Build history of the part. All positions in model axes, mm. Coordinates: 2 decimals unless noted, no trailing zeros. Write each loop counter-clockwise with the first axis right and the second up, starting at its lowest first coordinate (ties: lowest second). Pieces come first, ordered by that corner, then holes. Notation, with made-up numbers: (62.5, 83.5) -> (109.5, 83.5) arc R29 ccw to (109.5, 121.5) -> close; hole circle Ø3 at (73.25, -3.75). An arc over 180 degrees is marked (long way). Write each question's results on one line, items separated by ' | '. Start each with the question number.
Q1. Drill centre lines: line 1 (Y direction, x = 78.5, z = 0.75); line 2 (Y direction, x = -36.5, z = 0.75); line 3 (X direction, y = 98, z = 4). Where is each one in solid material? Low to high.
Q2. Saw through at A-A on y = -14. Give the cut face in (x, z).
Q3. Saw through at B-B on x = 72.5. Give the cut face in (y, z).
Q4. Saw through at C-C on y = 35. Give the cut face in (x, z).
Q5. Two-plate mould, pull along Y, no slides. Class faces 1 (the face through (61, 25.4, 3)), 2 (the face through (139.203, 123.181, 3.131)), 3 (the face through (-139.203, -123.181, 3.131)), 4 (the face through (-90, -120.694, 3)): released by +Y, released by -Y, zero draft, split by the parting line, or undercut.
Q6. Drop flat-ended pins along their axis: pin 1 Ø3 at (y, z) = (118.5, 4) entering from +X; pin 2 Ø3 at (y, z) = (-118, 2) entering from +X; pin 3 Ø1.9 at (y, z) = (-118, 4) entering from -X. Give the stop position or say it passes through.
Q7. Saw through at D-D on x = -14. Give the cut face in (y, z).
from build123d import *

# Parameters (mm, degrees)
F0_W     = 25.4
F0_H     = 6.35
F1_DEPTH = 6.35
F2_R     = 38.1


# Not quite as in the source:
# - a feature names something its author has since deleted; it is built from what else it names


with BuildPart() as f1:
    # F0 (on Top) → F1 (new body)
    with BuildSketch(Plane.XY):
        with BuildLine():
            ThreePointArc((142.8242, 114.3), (139.1044561211, 123.2802561211), (130.1242, 127))
            Line((130.1242, 127), (-130.1242, 127))
            ThreePointArc((-130.1242, 127), (-139.1044561211, 123.2802561211), (-142.8242, 114.3))
            Line((-142.8242, 114.3), (-142.8242, -114.3))
            ThreePointArc((-142.8242, -114.3), (-139.1044561211, -123.2802561211), (-130.1242, -127))
            Line((-130.1242, -127), (130.1242, -127))
            ThreePointArc((130.1242, -127), (139.1044561211, -123.2802561211), (142.8242, -114.3))
            Line((142.8242, -114.3), (142.8242, 114.3))
        make_face()
        with Locations((-90.0851422843, -117.5192241168)):
            Rectangle(F0_W, F0_H, mode=Mode.SUBTRACT)
        with Locations((-90.0684, -3.175)):
            Rectangle(F0_W, F0_H, mode=Mode.SUBTRACT)
        with Locations((90.0851422843, -117.5192241168)):
            Rectangle(F0_W, F0_H, mode=Mode.SUBTRACT)
        with Locations((90.0684, -3.175)):
            Rectangle(F0_W, F0_H, mode=Mode.SUBTRACT)
        with Locations((-90.0851422843, 117.5192241168)):
            Rectangle(F0_W, F0_H, mode=Mode.SUBTRACT)
        with BuildLine():
            Line((0, 101.6), (7.0708802395, 101.6))
            Line((7.0708802395, 101.6), (111.125, 101.6))
            ThreePointArc((111.125, 101.6), (114.3, 104.775), (117.475, 101.6))
            ThreePointArc((117.475, 101.6), (116.5450640303, 99.3549359697), (114.3, 98.425))
            Line((114.3, 98.425), (114.3, 25.4))
            Line((114.3, 25.4), (44.3961802395, 25.4))
            Line((44.3961802395, 25.4), (37.3253, 25.4))
            Line((37.3253, 25.4), (37.3253, -25.4))
            Line((37.3253, -25.4), (44.3961802395, -25.4))
            Line((44.3961802395, -25.4), (114.3, -25.4))
            Line((114.3, -25.4), (114.3, -98.425))
            ThreePointArc((114.3, -98.425), (116.5450640303, -99.3549359697), (117.475, -101.6))
            ThreePointArc((117.475, -101.6), (114.3, -104.775), (111.125, -101.6))
            Line((111.125, -101.6), (7.0708802395, -101.6))
            Line((7.0708802395, -101.6), (0, -101.6))
            Line((0, -101.6), (-7.0708802395, -101.6))
            Line((-7.0708802395, -101.6), (-111.125, -101.6))
            ThreePointArc((-111.125, -101.6), (-116.5450640303, -103.8450640303), (-114.3, -98.425))
            Line((-114.3, -98.425), (-114.3, -25.4))
            Line((-114.3, -25.4), (-44.3961802395, -25.4))
            Line((-44.3961802395, -25.4), (-37.3253, -25.4))
            Line((-37.3253, -25.4), (-37.3253, 25.4))
            Line((-37.3253, 25.4), (-44.3961802395, 25.4))
            Line((-44.3961802395, 25.4), (-114.3, 25.4))
            Line((-114.3, 25.4), (-114.3, 98.425))
            ThreePointArc((-114.3, 98.425), (-116.5450640303, 103.8450640303), (-111.125, 101.6))
            Line((-111.125, 101.6), (-7.0708802395, 101.6))
            Line((-7.0708802395, 101.6), (0, 101.6))
        make_face(mode=Mode.SUBTRACT)
        with Locations((90.0851422843, 117.5192241168)):
            Rectangle(F0_W, F0_H, mode=Mode.SUBTRACT)
        Polygon((-37.3253, 25.4), (0, 101.6), (-7.0708802395, 101.6), (-44.3961802395, 25.4), align=None)
        Polygon((44.3961802395, 25.4), (7.0708802395, 101.6), (0, 101.6), (37.3253, 25.4), align=None)
        Polygon((44.3961802395, -25.4), (37.3253, -25.4), (0, -101.6), (7.0708802395, -101.6), align=None)
        Polygon((0, -101.6), (-37.3253, -25.4), (-44.3961802395, -25.4), (-7.0708802395, -101.6), align=None)
    extrude(amount=F1_DEPTH)

    # F2
    f2_edges = [f1.edges().sort_by_distance(p)[0] for p in [
        (7.07088, 101.6, 3.175),
        (-7.07088, 101.6, 3.175),
        (114.3, 25.4, 3.175),
        (-114.3, 25.4, 3.175),
        (-114.3, -25.4, 3.175),
        (114.3, -25.4, 3.175),
        (-7.07088, -101.6, 3.175),
        (7.07088, -101.6, 3.175),
        (-114.3, 98.425, 3.175),
        (-111.125, 101.6, 3.175),
        (111.125, 101.6, 3.175),
        (114.3, 98.425, 3.175),
        (114.3, -98.425, 3.175),
        (111.125, -101.6, 3.175),
        (-111.125, -101.6, 3.175),
        (-114.3, -98.425, 3.175),
    ]]
    fillet(f2_edges, radius=F2_R)


solid = f1.part
Returned:
1) line 1: y = -127 to -120.69, -114.34 to -101.6, -25.47 to -6.35, 0 to 25.47, 101.6 to 114.34, 120.69 to 127 | line 2: y = -127 to -84.7, -41.52 to -27.08, 27.08 to 41.52, 84.7 to 127 | line 3: x = -142.82 to -116.33, -51.99 to -1.76, 1.76 to 51.99, 116.33 to 142.82
2) outline: (-142.82, 0) -> (-37.33, 0) -> (-37.33, 6.35) -> (-142.82, 6.35) -> close; (37.33, 0) -> (142.82, 0) -> (142.82, 6.35) -> (37.33, 6.35) -> close
3) outline: (-127, 0) -> (-101.6, 0) -> (-101.6, 6.35) -> (-127, 6.35) -> close; (-25.4, 0) -> (25.4, 0) -> (25.4, 6.35) -> (-25.4, 6.35) -> close; (101.6, 0) -> (127, 0) -> (127, 6.35) -> (101.6, 6.35) -> close
4) outline: (-142.82, 0) -> (-101.49, 0) -> (-101.49, 6.35) -> (-142.82, 6.35) -> close; (-39.69, 0) -> (-32.62, 0) -> (-32.62, 6.35) -> (-39.69, 6.35) -> close; (32.62, 0) -> (39.69, 0) -> (39.69, 6.35) -> (32.62, 6.35) -> close; (101.49, 0) -> (142.82, 0) -> (142.82, 6.35) -> (101.49, 6.35) -> close
5) face 1: undercut | face 2: released by +Y | face 3: released by -Y | face 4: undercut
6) pin 1: stops at x = 142.53 | pin 2: stops at x = 142.63 | pin 3: stops at x = -142.52
7) outline: (-127, 0) -> (-73.02, 0) -> (-73.02, 6.35) -> (-127, 6.35) -> close; (73.02, 0) -> (127, 0) -> (127, 6.35) -> (73.02, 6.35) -> close
